```python
from build123d import *

# Parameters (mm, degrees)
BOSS_EXTRUDE2_DEPTH = 10
SKETCH2_R           = 7
CUT_EXTRUDE1_DEPTH  = 21.880613018
SKETCH3_OUTSIDE_W   = 68.242
SKETCH3_OUTSIDE_H   = 71.954
SKETCH3_OUTSIDE_R   = 12
CUT_EXTRUDE2_DEPTH  = 10
CUT_EXTRUDE2_DRAFT  = -60
SKETCH4_OUTSIDE_W   = 68.242
SKETCH4_OUTSIDE_H   = 71.954
SKETCH4_OUTSIDE_R   = 12
CUT_EXTRUDE3_DEPTH  = 10
CUT_EXTRUDE3_DRAFT  = -60
CHAMFER1_SIZE       = 1


with BuildPart() as part:
    # Sketch1 → Boss-Extrude2 (new body)
    with BuildSketch(Plane.XY):
        Polygon((12, -6.92820323), (12, 6.92820323), (0, 13.856406461), (-12, 6.92820323), (-12, -6.92820323), (0, -13.856406461), align=None)
    extrude(amount=BOSS_EXTRUDE2_DEPTH)

    # Sketch2 → Cut-Extrude1 (cut, through all)
    with BuildSketch(Plane.XY.offset(10)):
        Circle(SKETCH2_R)
    extrude(amount=-CUT_EXTRUDE1_DEPTH, mode=Mode.SUBTRACT)


with BuildPart() as cut_extrude2_tool:
    # Sketch3 outside → Cut-Extrude2 (with draft: the straight prism first)
    with BuildSketch(Plane.XY.offset(10)):
        Rectangle(SKETCH3_OUTSIDE_W, SKETCH3_OUTSIDE_H)
        Circle(SKETCH3_OUTSIDE_R, mode=Mode.SUBTRACT)
    extrude(amount=-CUT_EXTRUDE2_DEPTH)
    # Cut-Extrude2: the draft: its side faces are tilted about the plane it starts from
    cut_extrude2_sides = [cut_extrude2_tool.faces().sort_by_distance(p)[0] for p in [
        (0, -35.977, 5),
        (34.121, 0, 5),
        (0, 35.977, 5),
        (-34.121, 0, 5),
        (-12, 0, 5),
    ]]
    draft(cut_extrude2_sides, Plane.XY.offset(10), CUT_EXTRUDE2_DRAFT)


with BuildPart() as part_1:
    add(part.part)

    # Cut-Extrude2: cut by cut_extrude2_tool
    add(cut_extrude2_tool.part, mode=Mode.SUBTRACT)


with BuildPart() as cut_extrude3_tool:
    # Sketch4 outside → Cut-Extrude3 (with draft: the straight prism first)
    with BuildSketch(Plane(origin=(0, 0, 0), x_dir=(-1, 0, 0), z_dir=(0, 0, -1))):
        Rectangle(SKETCH4_OUTSIDE_W, SKETCH4_OUTSIDE_H)
        Circle(SKETCH4_OUTSIDE_R, mode=Mode.SUBTRACT)
    extrude(amount=-CUT_EXTRUDE3_DEPTH)
    # Cut-Extrude3: the draft: its side faces are tilted about the plane it starts from
    cut_extrude3_sides = [cut_extrude3_tool.faces().sort_by_distance(p)[0] for p in [
        (0, -35.977, 5),
        (-34.121, 0, 5),
        (0, 35.977, 5),
        (34.121, 0, 5),
        (12, 0, 5),
    ]]
    draft(cut_extrude3_sides, Plane(origin=(0, 0, 0), x_dir=(-1, 0, 0), z_dir=(0, 0, -1)), CUT_EXTRUDE3_DRAFT)


with BuildPart() as part_2:
    add(part_1.part)

    # Cut-Extrude3: cut by cut_extrude3_tool
    add(cut_extrude3_tool.part, mode=Mode.SUBTRACT)

    # Chamfer1
    chamfer1_edges = [part_2.edges().sort_by_distance(p)[0] for p in [
        (-7, 0, 0),
        (-7, 0, 10),
    ]]
    chamfer(chamfer1_edges, length=CHAMFER1_SIZE)


solid = part_2.part
```
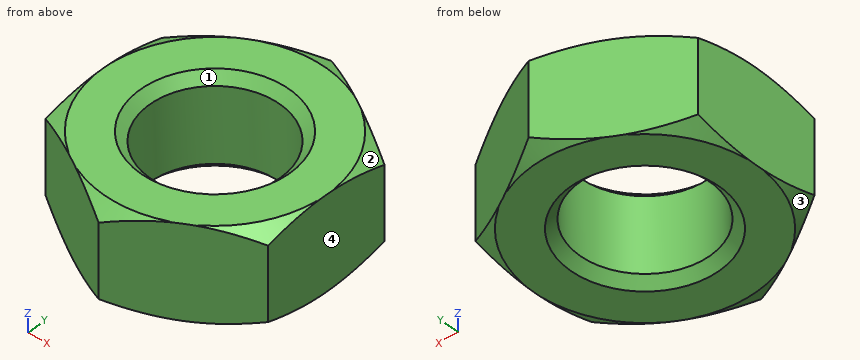
Check sheet for the modelled part. Datum: model origin and axes. Units: mm. Face numbers are marked on the shaded views. Round coordinates to 2 decimals unless told otherwise and drop trailing zeros. Order: outer loops, then holes, each group sorted by start corner. A loop starts at its lowest first (then second) coordinate and runs counter-clockwise, first axis right, second up.
1) Go/stop test with a flat-tipped pin: pin 1 Ø3 at (x, z) = (6.5, 1.5) entering from +Y. Record where the tip stops, or that it passes through.
2) Mould release check, pull along Y, two halves, no side actions. Record for the marked faces 1, 2, 3 and 4: +Y half, -Y half, draft (parallel to the pull), parting line (faces both ways), or undercut.
3) Section check A-A (z = 1.5). Record the boundary of the cut face in (x, y).
4) Scan lines: line 1 (Y direction, x = 2, z = 3.25); line 2 (Y direction, x = 3.25, z = 6.25); line 3 (X direction, y = -3.25, z = 6). Record each from-to range of solid material in increasing order.
Result:
1. pin 1: stops at y = 10.97
2. face 1: undercut
2. face 2: +Y half
2. face 3: -Y half
2. face 4: draft
3. outline: (-12, -6.93) - (0, -13.86) - (12, -6.93) - (12, 6.93) - (0, 13.86) - (-12, 6.93) - close; hole circle Ø14 at (0, 0)
4. line 1: y = -12.7 to -6.71, 6.71 to 12.7
4. line 2: y = -11.98 to -6.2, 6.2 to 11.98
4. line 3: x = -12 to -6.2, 6.2 to 12
